Answer from the drawing. Dimensions are ordinates in mm from the lowest x, y and z of the part. A direction names the side the tool comes from. Coordinates: 2 decimals unless noted, no trailing zeros. Loops run counter-clockwise (first coordinate to the right, second up) from the corner with the lowest first, then second, coordinate; pieces in that order, holes last. Notation, with made-up numbers: (-7.75, 80.25) - (7.25, 80.25) arc R10 cw to (7.25, 91.25) - close; hole circle Ø11 at (-34, -7). An arc over 180 degrees is marked (long way). Use one line per item in the form item = value. Start each with the question number.
1) A cutting plane is placed at B-B (x = 53). Give the vertices of the cut face in (y, z) (1 decimal), and give its area (3 significant figures).
2) A cutting plane is placed at D-D (y = 18.5). Give the vertices of the cut face in (x, z) (1 decimal), and give its area (3 significant figures).
3) A cutting plane is placed at C-C (z = 50). Give the vertices of the cut face in (x, y) (1 decimal).
4) Each of these flat-tipped pins is pushed along its axis until it touches: P1, Ø5, axis at y = 52, z = 95.5, coming from the -X side; P2, Ø4, axis at y = 20, z = 37.5, coming from the -X side; P3, Ø7.5, axis at x = 22, y = 50, coming from the +Z side; P4, Ø21.5, axis at x = 89.5, y = 33, coming from the +Z side. Where does it stop, or does it pass through?
5) Consider line 1 (X direction, y = 80.5, z = 74); line 2 (Z direction, x = 81, y = 22) (1 decimal); line 3 (Y direction, x = 49.5, z = 71). Determine where each line is inside the solid, lowest interval first.
6) A cutting plane is placed at A-A (y = 75.5). Give the vertices of the cut face in (x, z) (1 decimal), and give its area (3 significant figures).
7) Which of the six approach directions +Z, -Z, +X, -X, +Y, -Y give full straight-line access (tool end or side, diameter ignored) to the marked faces 1, 2, 3, 4 and 5?
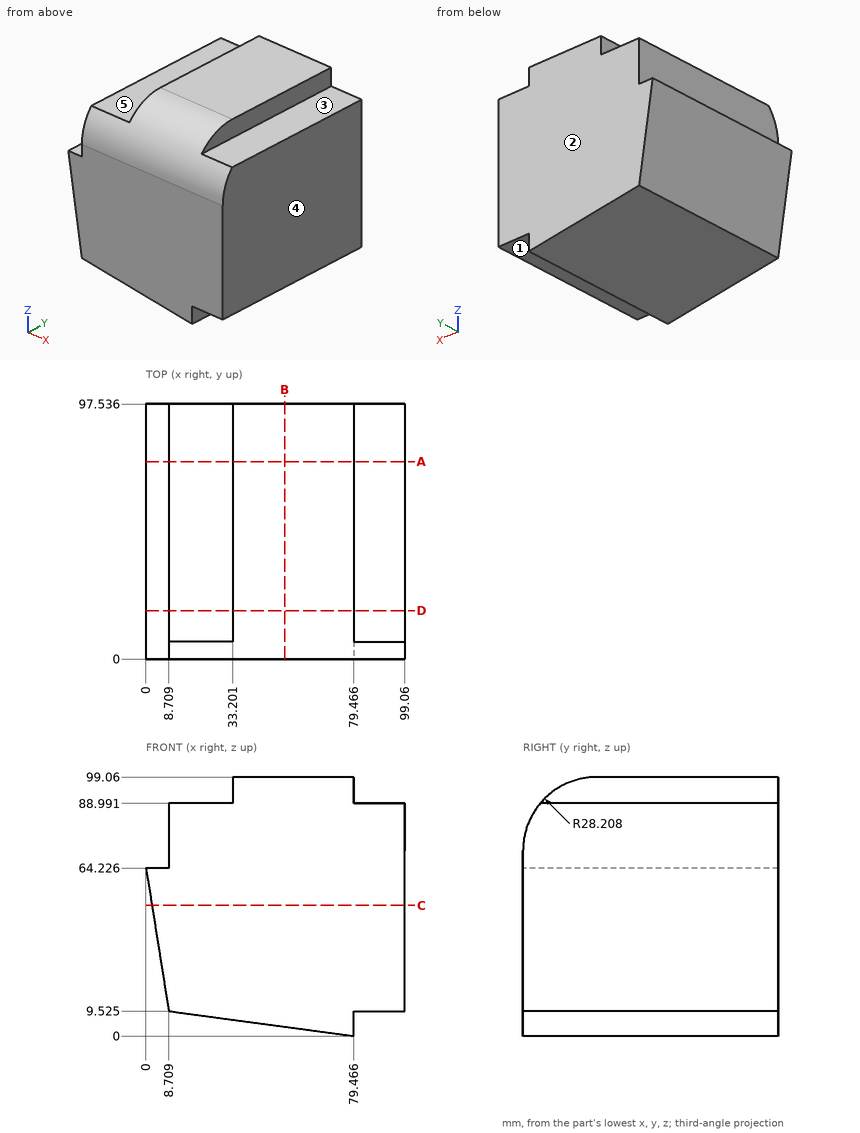
Found:
q1.outline = (0, 3.6) - (97.5, 3.6) - (97.5, 99.1) - (28.2, 99.1) arc R28.2 ccw to (0, 70.9) - close
q1.area = 9,140 mm^2
q2.outline = (0, 64.2) - (8.7, 9.5) - (79.5, 0) - (79.5, 9.5) - (99.1, 9.5) - (99.1, 89) - (79.5, 89) - (79.5, 97.3) - (33.2, 97.3) - (33.2, 89) - (8.7, 89) - (8.7, 64.2) - close
q2.area = 8,140 mm^2
q3.outline = (2.3, 0) - (99.1, 0) - (99.1, 97.5) - (2.3, 97.5) - close
q4.P1 = 33.2
q4.P2 = 3.94
q4.P3 = 88.99
q4.P4 = 99.06
q5.line_1 = 8.71 to 99.06
q5.line_2 = 9.5 to 89
q5.line_3 = 0 to 97.54
q6.outline = (0, 64.2) - (8.7, 9.5) - (79.5, 0) - (79.5, 9.5) - (99.1, 9.5) - (99.1, 89) - (79.5, 89) - (79.5, 99.1) - (33.2, 99.1) - (33.2, 89) - (8.7, 89) - (8.7, 64.2) - close
q6.area = 8,220 mm^2
q7.face_1 = -Z, +X, +Y, -Y
q7.face_2 = +Z, -Z, +X, -X, +Y
q7.face_3 = +Z, +X, +Y, -Y
q7.face_4 = +Z, -Z, +X, +Y, -Y
q7.face_5 = +Z, -X, +Y, -Y
